Verification items for the finished model (mm, model axes). A direction names the side the tool comes from. Round coordinates to 2 decimals unless told otherwise and drop trailing zeros. Loops run counter-clockwise (first coordinate to the right, second up) from the corner with the lowest first, then second, coordinate; pieces in that order, holes last. Notation, with made-up numbers: (65, -40) -> (105, -40) arc R26 ccw to (105, -7) -> close; hole circle Ø5 at (56, -30.75). An arc over 180 degrees is marked (long way). Write item = value, one per line.
```python
from build123d import *

# Parameters (mm, degrees)
SKETCH1_R                 = 1.5875
SKETCH1_W                 = 25.4
SKETCH1_H                 = 53.835078528
EXTRUDE1_DEPTH            = 9.525
FILLET1_R                 = 6.35
FILLET2_R                 = 6.35
CHAMFER3_SIZE             = 4.445
SKETCH2_R                 = 2.000000064
CUT_EXTRUDE1_DEPTH        = 91.671774296
SKETCH3_R                 = 1.016
CUT_EXTRUDE2_DEPTH        = 96.649297718
LPATTERN1_COUNT           = 3
LPATTERN1_PITCH           = 6.35
LPATTERN1_COPY_1_SKETCH_R = 1.016
LPATTERN1_COPY_1_DEPTH    = 96.649297718
LPATTERN1_COPY_2_SKETCH_R = 1.016
LPATTERN1_COPY_2_DEPTH    = 96.649297718


with BuildPart() as part:
    # Sketch1 → Extrude1 (new body)
    with BuildSketch(Plane.XY):
        Polygon((57.023, 60.185078528), (57.023, 76.2), (-57.023, 76.2), (-57.023, 60.185078528), (-19.05, 60.185078528), (-19.05, 6.35), (-38.1, 6.35), (-38.1, 0), (38.1, 0), (38.1, 6.35), (19.05, 6.35), (19.05, 60.185078528), align=None)
        with Locations((-49.403, 68.58)):
            Circle(SKETCH1_R, mode=Mode.SUBTRACT)
        with Locations((49.403, 68.58)):
            Circle(SKETCH1_R, mode=Mode.SUBTRACT)
        with Locations((0, 33.267539264)):
            Rectangle(SKETCH1_W, SKETCH1_H, mode=Mode.SUBTRACT)
    extrude(amount=-EXTRUDE1_DEPTH)

    # Fillet1
    fillet1_edges = [part.edges().sort_by_distance(p)[0] for p in [
        (-57.023, 60.185078528, -4.7625),
        (-57.023, 76.2, -4.7625),
        (57.023, 76.2, -4.7625),
        (57.023, 60.185078528, -4.7625),
    ]]
    fillet(fillet1_edges, radius=FILLET1_R)

    # Fillet2
    fillet2_edges = [part.edges().sort_by_distance(p)[0] for p in [
        (-19.05, 6.35, -4.7625),
        (-19.05, 60.185078528, -4.7625),
        (19.05, 60.185078528, -4.7625),
        (19.05, 6.35, -4.7625),
        (-12.7, 60.185078528, -4.7625),
        (12.7, 60.185078528, -4.7625),
        (12.7, 6.35, -4.7625),
        (-12.7, 6.35, -4.7625),
    ]]
    fillet(fillet2_edges, radius=FILLET2_R)

    # Chamfer3
    # the kernel refuses this chamfer: 4.445 mm, written as the material it takes off along each edge
    with BuildSketch(Plane(origin=(50.673, 76.2, 0), x_dir=(0, -0.9996219169112966, 0.02749587661058641), z_dir=(-1, 0, 0))) as chamfer3_piece_1:
        Polygon((CHAMFER3_SIZE * 0.999621916911, -CHAMFER3_SIZE * 0.0274958766106), (-CHAMFER3_SIZE * 0.0274958766106, -CHAMFER3_SIZE * 0.999621916911), (0, 0), align=None)
    extrude(amount=101.346, mode=Mode.SUBTRACT)
    with BuildSketch(Plane(origin=(57.023, 66.535078528, 0), x_dir=(-0.9996219169112966, 0, 0.027495876610586344), z_dir=(0, 1, 0)), Plane(origin=(-57.023, 69.85, 0), x_dir=(0.9996219169112966, 0, 0.027495876610586344), z_dir=(0, -1, 0))) as chamfer3_piece_2:
        Polygon((CHAMFER3_SIZE * 0.999621916911, -CHAMFER3_SIZE * 0.0274958766106), (-CHAMFER3_SIZE * 0.0274958766106, -CHAMFER3_SIZE * 0.999621916911), (0, 0), align=None)
    extrude(amount=3.314921472, mode=Mode.SUBTRACT)
    with BuildSketch(Plane(origin=(-50.673, 60.185078528, 0), x_dir=(0, 0.9996219169112966, 0.027495876610586344), z_dir=(1, 0, 0)), Plane(origin=(25.4, 60.185078528, 0), x_dir=(0, 0.9996219169112966, 0.02749587661058641), z_dir=(1, 0, 0))) as chamfer3_piece_3:
        Polygon((CHAMFER3_SIZE * 0.999621916911, -CHAMFER3_SIZE * 0.0274958766106), (-CHAMFER3_SIZE * 0.0274958766106, -CHAMFER3_SIZE * 0.999621916911), (0, 0), align=None)
    extrude(amount=25.273, mode=Mode.SUBTRACT)
    with BuildSketch(Plane(origin=(50.673, 66.535078528, 0), x_dir=(1, 0, 0), z_dir=(0, 1, 0))) as chamfer3_piece_4:
        Polygon((6.35 - CHAMFER3_SIZE, 0), (6.35, CHAMFER3_SIZE), (6.35, 0), align=None)
    revolve(axis=Axis((50.673, 66.535078528, 0), (0, 0, -1)), revolution_arc=90, mode=Mode.SUBTRACT)
    with BuildSketch(Plane(origin=(-50.673, 66.535078528, 0), x_dir=(-1, 0, 0), z_dir=(0, 1, 0))) as chamfer3_piece_5:
        Polygon((6.35 - CHAMFER3_SIZE, 0), (6.35, -CHAMFER3_SIZE), (6.35, 0), align=None)
    revolve(axis=Axis((-50.673, 66.535078528, 0), (0, 0, 1)), revolution_arc=90, mode=Mode.SUBTRACT)
    with BuildSketch(Plane(origin=(50.673, 69.85, 0), x_dir=(1, 0, 0), z_dir=(0, -1, 0))) as chamfer3_piece_6:
        Polygon((6.35 - CHAMFER3_SIZE, 0), (6.35, -CHAMFER3_SIZE), (6.35, 0), align=None)
    revolve(axis=Axis((50.673, 69.85, 0), (0, 0, 1)), revolution_arc=90, mode=Mode.SUBTRACT)
    with BuildSketch(Plane(origin=(-50.673, 69.85, 0), x_dir=(0, 1, 0), z_dir=(1, 0, 0))) as chamfer3_piece_7:
        Polygon((6.35 - CHAMFER3_SIZE, 0), (6.35, -CHAMFER3_SIZE), (6.35, 0), align=None)
    revolve(axis=Axis((-50.673, 69.85, 0), (0, 0, 1)), revolution_arc=90, mode=Mode.SUBTRACT)
    with BuildSketch(Plane(origin=(25.4, 53.835078528, 0), x_dir=(0, 1, 0), z_dir=(1, 0, 0))) as chamfer3_piece_8:
        Polygon((6.35 + CHAMFER3_SIZE, 0), (6.35, -CHAMFER3_SIZE), (6.35, 0), align=None)
    revolve(axis=Axis((25.4, 53.835078528, 0), (0, 0, 1)), revolution_arc=193.184040246, mode=Mode.SUBTRACT)
    with BuildSketch(Plane(origin=(-25.4, 53.835078528, 0), x_dir=(0, 1, 0), z_dir=(-1, 0, 0))) as chamfer3_piece_9:
        Polygon((6.35 + CHAMFER3_SIZE, 0), (6.35, CHAMFER3_SIZE), (6.35, 0), align=None)
    revolve(axis=Axis((-25.4, 53.835078528, 0), (0, 0, -1)), revolution_arc=193.184040246, mode=Mode.SUBTRACT)

    # Sketch2 → Cut-Extrude1 (cut, through all)
    with BuildSketch(Plane(origin=(0, 6.35, 0), x_dir=(1, 0, 0), z_dir=(0, 1, 0))):
        with Locations(Location((31.410975272, 4.7625, 0), (0, 0, 270))):
            Circle(SKETCH2_R)
    cut_extrude1 = extrude(amount=-CUT_EXTRUDE1_DEPTH, mode=Mode.SUBTRACT)

    # Mirror1: Cut-Extrude1 across plane
    add(cut_extrude1.mirror(Plane(origin=(0, 0, 0), x_dir=(0, 0, 1), z_dir=(1, 0, 0))), mode=Mode.SUBTRACT)

    # Sketch3 → Cut-Extrude2 (cut, through all)
    with BuildSketch(Plane.XY):
        with Locations((16.002, 25.4)):
            Circle(SKETCH3_R)
    cut_extrude2 = extrude(amount=-CUT_EXTRUDE2_DEPTH, mode=Mode.SUBTRACT)

    # Mirror2: Cut-Extrude2 across plane
    add(cut_extrude2.mirror(Plane(origin=(0, 0, 0), x_dir=(0, 0, 1), z_dir=(1, 0, 0))), mode=Mode.SUBTRACT)

    # LPattern1: Cut-Extrude2 ×3
    with Locations(*[(0, -i * LPATTERN1_PITCH, 0) for i in range(1, LPATTERN1_COUNT)]):
        add(cut_extrude2, mode=Mode.SUBTRACT)

    # LPattern1 copy 1 sketch → LPattern1 copy 1 (cut, through all)
    with BuildSketch(Plane(origin=(0, -6.35, 0), x_dir=(-1, 0, 0), z_dir=(0, 0, 1))):
        with Locations((16.002, -25.4)):
            Circle(LPATTERN1_COPY_1_SKETCH_R)
    extrude(amount=-LPATTERN1_COPY_1_DEPTH, mode=Mode.SUBTRACT)

    # LPattern1 copy 2 sketch → LPattern1 copy 2 (cut, through all)
    with BuildSketch(Plane(origin=(0, -12.7, 0), x_dir=(-1, 0, 0), z_dir=(0, 0, 1))):
        with Locations((16.002, -25.4)):
            Circle(LPATTERN1_COPY_2_SKETCH_R)
    extrude(amount=-LPATTERN1_COPY_2_DEPTH, mode=Mode.SUBTRACT)


solid = part.part
```
(1) Material ranges on probe 1 along X at (y, z) = (68.5, -6.25); probe 2 along X at (y, z) = (45, -6.5); probe 3 along Y at (x, z) = (-2, -8.25), recorded low to high. Write a range as from..to.
Filled sheet:
probe_1 = -57.02..-50.99, -47.82..47.82, 50.99..57.02
probe_2 = -19.05..-12.7, 12.7..19.05
probe_3 = 0..6.35, 60.19..76.2
(2) Go/stop test with flat-tipped pins: pin 1 Ø2.5 at (x, y) = (-16.002, 12.7) entering from +Z; pin 2 Ø1 at (y, z) = (55, -7) entering from -X; pin 3 Ø5 at (y, z) = (30, -4) entering from +X; pin 4 Ø1.2 at (x, y) = (16.002, 12.7) entering from +Z. Record where each tip stops, or that it passes through.
Filled sheet:
pin_1 = 0
pin_2 = -19.27
pin_3 = 19.05
pin_4 = through
(3) Draft check along Y on faces 5 (the face through (38.1, 3, -5)), 6 (the face through (-1, 0, -5)), 7 (the face through (-19.05, 34, -5)). Enter one of: released by +Y, released by -Y, zero draft, split by the parting line, or undercut.
Filled sheet:
face_5 = zero draft
face_6 = released by -Y
face_7 = undercut
(4) Sectioned sample at D-D, the plane y = 9. Record the cut outline in (x, z) (3 decimals), and give its area (3 significant figures).
Filled sheet:
outline = (-20.239, -9.525) -> (-11.511, -9.525) -> (-11.511, 0) -> (-20.239, 0) -> close; (11.511, -9.525) -> (20.239, -9.525) -> (20.239, 0) -> (11.511, 0) -> close
area = 166 mm2
(5) Sectioned sample at A-A, the plane y = 33. Record the cut outline in (x, z) (3 decimals), and give its area (3 significant figures).
Filled sheet:
outline = (-19.05, -9.525) -> (-12.7, -9.525) -> (-12.7, 0) -> (-19.05, 0) -> close; (12.7, -9.525) -> (19.05, -9.525) -> (19.05, 0) -> (12.7, 0) -> close
area = 121 mm2
(6) Sectioned sample at C-C, the plane y = 68.58. Record the cut outline in (x, z) (1 decimal).
Filled sheet:
outline = (-57, -9.5) -> (-51, -9.5) -> (-51, 0) -> (-52.6, 0) -> (-57, -4.4) -> close; (-47.8, -9.5) -> (47.8, -9.5) -> (47.8, 0) -> (-47.8, 0) -> close; (51, -9.5) -> (57, -9.5) -> (57, -4.4) -> (52.6, 0) -> (51, 0) -> close
(7) Sectioned sample at B-B, the plane x = 1. Record the cut outline in (y, z) (3 decimals).
Filled sheet:
outline = (0, -9.525) -> (6.35, -9.525) -> (6.35, 0) -> (0, 0) -> close; (60.185, -9.525) -> (76.2, -9.525) -> (76.2, -4.445) -> (71.755, 0) -> (60.185, 0) -> close
(8) Set-up check for faces 1 (the face through (20.86, 8.26, -4.83)), 2 (the face through (33.394, 3.219, -5.023)), 3 (the face through (0, 6.35, -5)), 4 (the face through (-38.21, 62.44, -2.19)): record each of +Z, -Z, +X, -X, +Y, -Y from which the full face is reachable in a straight line by a thin tool's end or side.
Filled sheet:
face_1 = +Z, -Z, +X
face_2 = -Y
face_3 = +Z, -Z
face_4 = +Z, -X
